Here's how the part is built. I have some questions about the finished solid (model axes, mm). Face numbers are marked on the shaded views. A direction names the side the tool comes from. Coordinates: 2 decimals unless noted, no trailing zeros. Loops run counter-clockwise (first coordinate to the right, second up) from the corner with the lowest first, then second, coordinate; pieces in that order, holes last. Notation, with made-up numbers: (-26.5, -32) -> (-12.5, -32) arc R26 cw to (-12.5, -5) -> close; hole circle Ø1 at (21.25, -23). An arc over 180 degrees is marked (long way). Use CSV: the item, a comma, the result in double quotes. Start each with the question number.
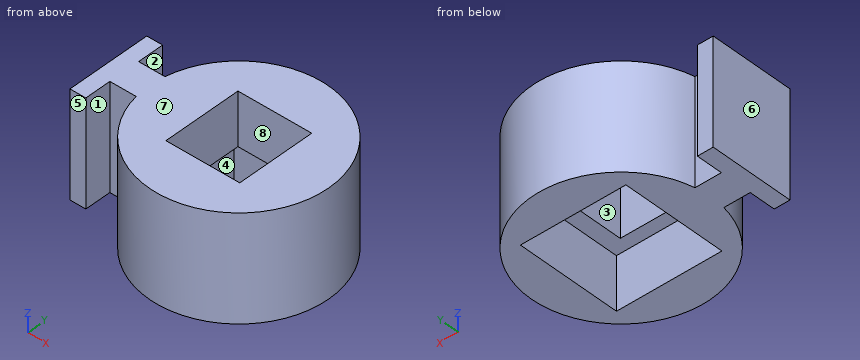
from build123d import *

# Parameters (mm, degrees)
PAD007_DEPTH            = 20
SKETCH018_W             = 15
SKETCH018_H             = 14
POCKET008_DEPTH         = 20.001
SKETCH019_W             = 20
SKETCH019_H             = 20
POCKET009_DEPTH         = 10.001
BODY006_PLACEMENT_ANGLE = 90


with BuildPart() as part:
    # Sketch017 → Pad007 (new body)
    with BuildSketch(Plane.XY):
        with BuildLine():
            Line((-3, -3), (-8, -3))
            Line((-8, -3), (-8, 0))
            Line((-8, 0), (8, 0))
            Line((8, 0), (8, -3))
            Line((8, -3), (3, -3))
            Line((3, -3), (3, -8))
            ThreePointArc((-3, -8), (0, -41.733201), (3, -8))
            Line((-3, -3), (-3, -8))
        make_face()
    extrude(amount=PAD007_DEPTH)

    # Sketch018 (on Face10 of Pad007) → Pocket008 (cut, through all)
    with BuildSketch(Plane.XY.offset(20)):
        with Locations((0, -24.733201)):
            Rectangle(SKETCH018_W, SKETCH018_H)
    extrude(amount=-POCKET008_DEPTH, mode=Mode.SUBTRACT)

    # Sketch019 (on Face5 of Pocket008) → Pocket009 (cut, through all)
    with BuildSketch(Plane.XY.offset(10)):
        with Locations((0, -24.733201)):
            Rectangle(SKETCH019_W, SKETCH019_H)
    extrude(amount=-POCKET009_DEPTH, mode=Mode.SUBTRACT)


with BuildPart() as part_1:
    # Body006 placement: moved
    add(part.part.moved(Location((32.5, 0, 180))).rotate(Axis((32.5, 0, 180), (0, 0, 1)), BODY006_PLACEMENT_ANGLE))


solid = part_1.part
1) I want a section at C-C, the plane x = 63.5. Please give me the cut outline in (y, z).
2) I want a section at A-A, the plane y = 0. Please give me the cut outline in (x, z), plus the area to 3 significant figures.
3) Thinking about a two-plate mould opening in X: for the marked faces 6, 7 and 8, which applies, pulls with the +X half, pulls with the -X half, needs draft (parallel to the pull), parting line crosses it, or undercut?
4) For P1, Ø1.5, axis at x = 33.5, z = 188, coming from the +Y side; P2, Ø2.5, axis at y = 5, z = 191.5, coming from the +X side; P3, Ø10, axis at x = 67, z = 183.5, coming from the +Y side, each with a flat end and sliding along its axis, tell me the tip position at first contact or that it passes through.
5) Please list where these lines run through material, in increasing order: L1, parallel to X at y = -4.5, z = 196.5; L2, parallel to X at y = 4.5, z = 184.75; L3, parallel to Z at x = 66, y = -7. Write a range as [from, to].
6) I want a section at D-D, the plane y = -5.5. Please give me the cut outline in (x, z).
7) I want a section at B-B, the plane z = 198.25. Please give me the cut outline in (x, y), plus the area to 3 significant figures.
8) Which directions (+Z, -Z, +X, -X, +Y, -Y) give clear straight access to the entire face, cutting with the end or side of a thin tool? Please do the marked faces 1, 2, 3, 4 and 5.
Return value:
1,outline,"(-15.8, 180) -> (-10, 180) -> (-10, 190) -> (-7.5, 190) -> (-7.5, 200) -> (-15.8, 200) -> close; (7.5, 190) -> (10, 190) -> (10, 180) -> (15.8, 180) -> (15.8, 200) -> (7.5, 200) -> close"
2,outline,"(32.5, 180) -> (47.23, 180) -> (47.23, 190) -> (50.23, 190) -> (50.23, 200) -> (32.5, 200) -> close; (64.23, 190) -> (67.23, 190) -> (67.23, 180) -> (74.23, 180) -> (74.23, 200) -> (64.23, 200) -> close"
2,area,"495 mm²"
3,face 6,"pulls with the -X half"
3,face 7,"needs draft"
3,face 8,"undercut"
4,P1,"stops at y = 8"
4,P2,"stops at x = 73.81"
4,P3,"stops at y = 16.32"
5,L1,"x = [32.5, 35.5], [40.84, 50.23], [64.23, 73.63]"
5,L2,"x = [32.5, 35.5], [40.84, 47.23], [67.23, 73.63]"
5,L3,"z = [190, 200]"
6,outline,"(32.5, 180) -> (35.5, 180) -> (35.5, 200) -> (32.5, 200) -> close; (41.15, 180) -> (47.23, 180) -> (47.23, 190) -> (50.23, 190) -> (50.23, 200) -> (41.15, 200) -> close; (64.23, 190) -> (67.23, 190) -> (67.23, 180) -> (73.32, 180) -> (73.32, 200) -> (64.23, 200) -> close"
7,outline,"(32.5, -8) -> (35.5, -8) -> (35.5, -3) -> (40.5, -3) arc R17 ccw (long way) to (40.5, 3) -> (35.5, 3) -> (35.5, 8) -> (32.5, 8) -> close; hole (50.23, -7.5) -> (64.23, -7.5) -> (64.23, 7.5) -> (50.23, 7.5) -> close"
7,area,"775 mm²"
8,face 1,"+Z, -Z, -Y"
8,face 2,"+Z, -Z, +Y"
8,face 3,"+Z, -Z"
8,face 4,"-Z"
8,face 5,"+Z, -Z, -X, -Y"
